Drawing for the job (mm, zero at the part's lowest x, y, z). Round coordinates to 2 decimals unless told otherwise and drop trailing zeros. Loops run counter-clockwise (first coordinate to the right, second up) from the corner with the lowest first, then second, coordinate; pieces in that order, holes last.
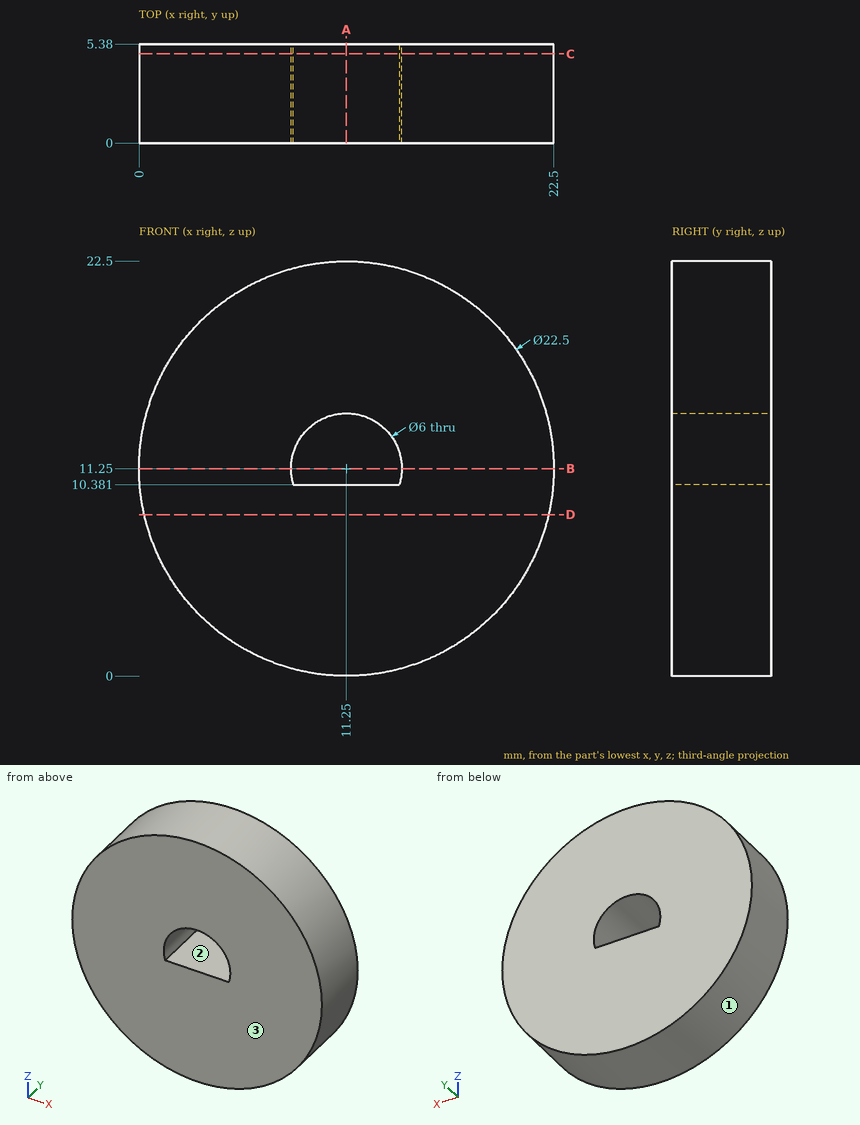
Q1. Slice it at B-B on z = 11.25. Give the cut face in (x, y).
Q2. Flat gauge pins, fed straight in: P1, Ø1, axis at x = 18.5, y = 1.5, coming from the +Z side; P2, Ø5, axis at x = 11.25, z = 11.25, coming from the +Y side; P3, Ø1, axis at y = 3.5, z = 13.5, coming from the +X side; P4, Ø1.5, axis at x = 10, y = 2, coming from the -Z side. Where does each tip first touch, or does it go through?
Q3. Slice it at D-D on z = 8.75. Give the cut face in (x, y), plus the area to 3 significant figures.
Q4. Slice it at C-C on y = 4.85. Give the cut face in (x, z).
Q5. Probe line 1 (Z direction, x = 11.25, y = 4); line 2 (X direction, y = 2.7, z = 11.25); line 3 (X direction, y = 3.85, z = 13) (1 decimal). List the from-to ranges inside material, lowest first.
Q6. Pull direction Z, two halves, no side cores. Call the marked faces 1, 2 and 3: pulls with the +Z half, pulls with the -Z half, needs draft (parallel to the pull), parting line crosses it, or undercut.
Q7. Slice it at A-A on x = 11.25. Give the cut face in (y, z), plus the area to 3 significant figures.
Reply:
1. outline: (0, 0) - (8.25, 0) - (8.25, 5.38) - (0, 5.38) - close; (14.25, 0) - (22.5, 0) - (22.5, 5.38) - (14.25, 5.38) - close
2. P1: stops at z = 20.25
2. P2: stops at y = 5.38
2. P3: stops at x = 22.36
2. P4: stops at z = 0.01
3. outline: (0.28, 0) - (22.22, 0) - (22.22, 5.38) - (0.28, 5.38) - close
3. area: 118 mm2
4. outline: circle Ø22.5 at (11.25, 11.25); hole (8.38, 10.38) - (14.12, 10.38) arc R3 ccw (long way) to start
5. line 1: z = 0 to 10.38, 14.25 to 22.5
5. line 2: x = 0 to 8.25, 14.25 to 22.5
5. line 3: x = 0.1 to 8.8, 13.7 to 22.4
6. face 1: parting line crosses it
6. face 2: undercut
6. face 3: needs draft
7. outline: (0, 0) - (5.38, 0) - (5.38, 10.38) - (0, 10.38) - close; (0, 14.25) - (5.38, 14.25) - (5.38, 22.5) - (0, 22.5) - close
7. area: 100 mm2
